For this review, take the finished solid that the model builds, in its own axes (mm). Face numbers are marked on the shaded views. A direction names the side the tool comes from. Coordinates: 2 decimals unless noted, no trailing zeros. Write each loop counter-clockwise with the first axis right and the second up, starting at its lowest first coordinate (ties: lowest second). Pieces come first, ordered by that corner, then holes.
```python
from build123d import *

# Parameters (mm, degrees)
BOSS_EXTRUDE1_DEPTH = 8
BOSS_EXTRUDE2_START = 8
BOSS_EXTRUDE2_DEPTH = 5
SKETCH5_W           = 4
SKETCH5_H           = 4
CUT_EXTRUDE1_DEPTH  = 8


with BuildPart() as part:
    # Sketch1 → Boss-Extrude1 (new body)
    with BuildSketch(Plane.XY):
        Polygon((9.375, -4.375), (9.375, -9.375), (4.375, -9.375), (-9.375, -9.375), (-9.375, 9.375), (9.375, 9.375), align=None)
    extrude(amount=BOSS_EXTRUDE1_DEPTH)

    # Sketch3 → Boss-Extrude2 (add)
    with BuildSketch(Plane.XY.offset(BOSS_EXTRUDE2_START)):
        Polygon((4.375, -9.375), (4.375, -29.375), (9.375, -29.375), (9.375, -9.375), (29.375, -9.375), (29.375, -4.375), (9.375, -4.375), (4.677094882, 0.322905118), (-0.322905118, -4.677094882), align=None)
    extrude(amount=BOSS_EXTRUDE2_DEPTH)

    # Sketch5 → Cut-Extrude1 (cut)
    with BuildSketch(Plane.XY):
        with Locations((7.375, -7.375)):
            Rectangle(SKETCH5_W, SKETCH5_H)
    extrude(amount=CUT_EXTRUDE1_DEPTH, mode=Mode.SUBTRACT)


solid = part.part
```
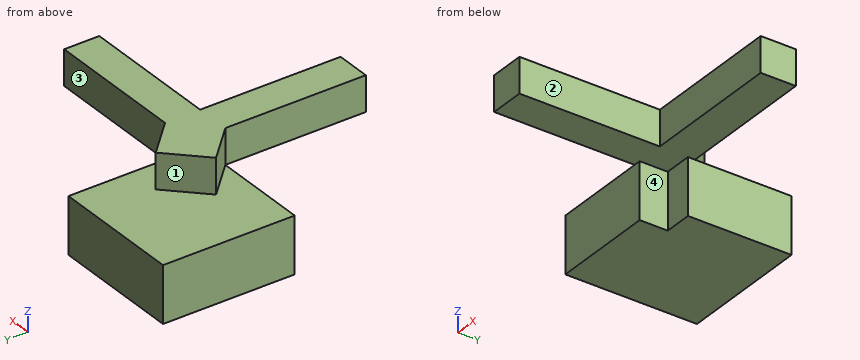
1) For L1, parallel to X at y = 5.5, z = 6.5 (3 decimals); L2, parallel to X at y = -25, z = 10.5 (3 decimals); L3, parallel to Z at x = -7, y = 5.5, list the stretches that pass through material, from the lowest coordinate up.
2) Consider section B-B (x = 8). Give the boundary of the cut face in (y, z) (3 decimals).
3) Clearance check with flat-ended pins moving along their axes: P1, Ø6, axis at x = 0.5, y = -12, coming from the +Z side; P2, Ø2.5, axis at x = -4.5, z = 3.5, coming from the -Y side (3 decimals); P3, Ø1, axis at x = 21, z = 10, coming from the +Y side (3 decimals). State where each tip first meets the part, or that it passes through.
4) Consider section A-A (y = -6). Give the boundary of the cut face in (x, z) (3 decimals), then the cut area to 3 significant figures.
5) Consider section D-D (z = 4.75). Give the boundary of the cut face in (x, y) (3 decimals), then the cut area to 3 significant figures.
6) Tool access review of the marked faces 1, 2, 3 and 4: name each direction out of +Z, -Z, +X, -X, +Y, -Y from which nothing blocks a thin tool from reaching the whole face with its end or side.
7) Consider section C-C (z = 11.5). Give the boundary of the cut face in (x, y) (3 decimals).
Results:
1. L1: x = -9.375 to 9.375
1. L2: x = 4.375 to 9.375
1. L3: z = 0 to 8
2. outline: (-29.375, 8) - (-5.375, 8) - (-5.375, 0) - (9.375, 0) - (9.375, 8) - (-3, 8) - (-3, 13) - (-29.375, 13) - close
3. P1: stops at z = 8
3. P2: stops at y = -9.375
3. P3: stops at y = -4.375
4. outline: (-9.375, 0) - (5.375, 0) - (5.375, 8) - (29.375, 8) - (29.375, 13) - (1, 13) - (1, 8) - (-9.375, 8) - close
4. area: 260 mm2
5. outline: (-9.375, -9.375) - (5.375, -9.375) - (5.375, -5.375) - (9.375, -5.375) - (9.375, 9.375) - (-9.375, 9.375) - close
5. area: 336 mm2
6. face 1: +Z, -X, +Y
6. face 2: +Z, -Z, +X, -Y
6. face 3: +Z, -Z, +X, +Y
6. face 4: -Z, +X, -Y
7. outline: (-0.323, -4.677) - (4.375, -9.375) - (4.375, -29.375) - (9.375, -29.375) - (9.375, -9.375) - (29.375, -9.375) - (29.375, -4.375) - (9.375, -4.375) - (4.677, 0.323) - close
